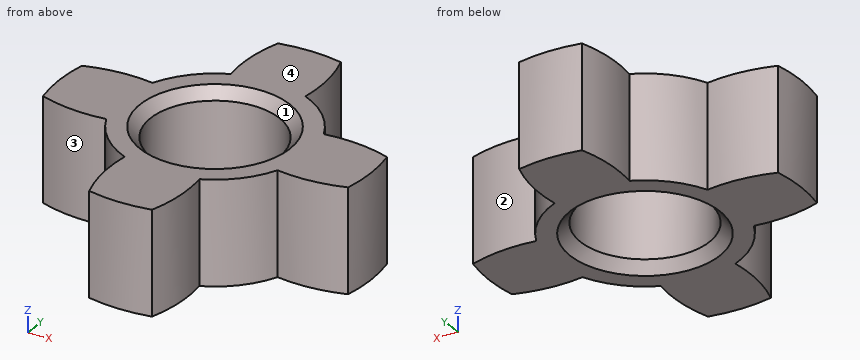
from build123d import *

# Parameters (mm, degrees)
SKETCH2_R          = 15
CUT_EXTRUDE1_DEPTH = 5


with BuildPart() as part:
    # Sketch1 → Revolve1 (revolve)
    with BuildSketch(Plane(origin=(0, 0, 0), x_dir=(0, 0, -1), z_dir=(1, 0, 0)), mode=Mode.PRIVATE) as revolve1_sk:
        Polygon((-5, 7.5), (-5, 3.6), (-4.5, 3.1), (-0.5, 3.1), (0, 3.6), (0, 7.5), align=None)
    revolve(revolve1_sk.sketch.rotate(Axis((0, 0, 0), (0, 0, 1)), 270), axis=Axis((0, 0, 0), (0, 0, 1)))

    # Sketch2 → Cut-Extrude1 (cut)
    with BuildSketch(Plane.XY):
        Circle(SKETCH2_R)
        with BuildLine():
            ThreePointArc((-9.892943155, 0), (-7.212770883, -1.555359899), (-4.123759488, -1.801279457))
            ThreePointArc((-4.123759488, -1.801279457), (-3.181980515, -3.181980515), (-1.801279457, -4.123759488))
            ThreePointArc((-1.801279457, -4.123759488), (-1.555359899, -7.212770883), (0, -9.892943155))
            ThreePointArc((0, -9.892943155), (1.555359899, -7.212770883), (1.801279457, -4.123759488))
            ThreePointArc((1.801279457, -4.123759488), (3.181980515, -3.181980515), (4.123759488, -1.801279457))
            ThreePointArc((4.123759488, -1.801279457), (7.212770883, -1.555359899), (9.892943155, 0))
            ThreePointArc((9.892943155, 0), (7.212770883, 1.555359899), (4.123759488, 1.801279457))
            ThreePointArc((4.123759488, 1.801279457), (3.181980515, 3.181980515), (1.801279457, 4.123759488))
            ThreePointArc((1.801279457, 4.123759488), (1.555359899, 7.212770883), (0, 9.892943155))
            ThreePointArc((0, 9.892943155), (-1.555359899, 7.212770883), (-1.801279457, 4.123759488))
            ThreePointArc((-1.801279457, 4.123759488), (-3.181980515, 3.181980515), (-4.123759488, 1.801279457))
            ThreePointArc((-4.123759488, 1.801279457), (-7.212770883, 1.555359899), (-9.892943155, 0))
        make_face(mode=Mode.SUBTRACT)
    extrude(amount=CUT_EXTRUDE1_DEPTH, mode=Mode.SUBTRACT)


solid = part.part
Could you check a few things on this model? Use its own coordinates, in mm. Face numbers are marked on the shaded views. Coordinates: 2 decimals unless noted, no trailing zeros. Order: outer loops, then holes, each group sorted by start corner. A loop starts at its lowest first (then second) coordinate and runs counter-clockwise, first axis right, second up. Notation, with made-up numbers: (-24.75, 22) -> (7.25, 22) arc R19 ccw to (7.25, 38) -> close; hole circle Ø4 at (-25.75, -15.5). An arc over 180 degrees is marked (long way). One line per item, written item: value. Start each with the question number.
1) Imagine slicing it at D-D on y = -5. List the corners of the cut face in (x, z) for me.
2) Imagine slicing it at B-B on y = 0. List the corners of the cut face in (x, z) for me, plus the area to 3 significant figures.
3) We'd pull the mould along Y, two halves only. Please class the marked faces 1, 2, 3 and 4: +Y half, -Y half, draft (parallel to the pull), parting line (faces both ways), or undercut.
4) I'm going to push flat-ended pins straight in: pin 1 (7 mm diameter, centred on x = 0, y = 0, fed in from -Z); pin 2 (3 mm diameter, centred on y = 5.5, z = 2, fed in from -X); pin 3 (5 mm diameter, centred on x = -3.5, y = 4.5, fed in from -Z). Where does each tip first touch, or does it pass through?
5) Imagine slicing it at A-A on z = 2.45. List the corners of the cut face in (x, y) for me, plus the area to 3 significant figures.
6) If I drill on L1, parallel to Y at x = -5, z = 3.55; L2, parallel to X at y = 2, z = 3.1, over which ranges is the centre line in solid material (lowest first)? Write a range as [from, to].
Answer list:
1. outline: (-1.87, 0) -> (1.87, 0) -> (1.87, 5) -> (-1.87, 5) -> close
2. outline: (-7.5, 0) -> (-3.6, 0) -> (-3.1, 0.5) -> (-3.1, 4.5) -> (-3.6, 5) -> (-7.5, 5) -> close; (3.1, 0.5) -> (3.6, 0) -> (7.5, 0) -> (7.5, 5) -> (3.6, 5) -> (3.1, 4.5) -> close
2. area: 43.5 mm2
3. face 1: undercut
3. face 2: +Y half
3. face 3: -Y half
3. face 4: draft
4. pin 1: stops at z = 0.1
4. pin 2: stops at x = -2.06
4. pin 3: stops at z = 0
5. outline: (-7.35, -1.51) arc R7 ccw to (-4.12, -1.8) arc R4.5 ccw to (-1.8, -4.12) arc R7 ccw to (-1.51, -7.35) arc R7.5 ccw to (1.51, -7.35) arc R7 ccw to (1.8, -4.12) arc R4.5 ccw to (4.12, -1.8) arc R7 ccw to (7.35, -1.51) arc R7.5 ccw to (7.35, 1.51) arc R7 ccw to (4.12, 1.8) arc R4.5 ccw to (1.8, 4.12) arc R7 ccw to (1.51, 7.35) arc R7.5 ccw to (-1.51, 7.35) arc R7 ccw to (-1.8, 4.12) arc R4.5 ccw to (-4.12, 1.8) arc R7 ccw to (-7.35, 1.51) arc R7.5 ccw to start; hole circle Ø6.2 at (0, 0)
5. area: 77.0 mm2
6. L1: y = [-1.87, 1.87]
6. L2: x = [-4.03, -2.37], [2.37, 4.03]
